```python
from build123d import *

# Parameters (mm, degrees)
F1_DEPTH = 7.2


with BuildPart() as f1:
    # F0 (on Top) → F1 (new body)
    with BuildSketch(Plane.XY):
        with BuildLine():
            Line((-8.2668317482, -17.3311792314), (0.1017643333, -17.3311792314))
            Line((0.1017643333, -17.3311792314), (8.2668317482, -17.3311792314))
            add(Edge.make_bspline(
                [(36.6192528714, -21.1421355028), (36.0259011039, -22.4667622734), (33.1013576776, -26.9667648317), (23.9156707234, -28.3936125615), (14.039303545, -21.4118387937), (8.2668317482, -17.3311792314)],
                knots=[0.4597765415, 0.4597765415, 0.4597765415, 0.4597765415, 0.5296754291, 0.7251078993, 1, 1, 1, 1], degree=3))
            add(Edge.make_bspline(
                [(36.6192528714, -21.1421355028), (37.4697374215, -19.9659644134), (39.9045822409, -15.1832342327), (36.5474251452, -6.5147721142), (25.5628481096, -1.4524741246), (19.142657366, 1.506303313)],
                knots=[0.4597765415, 0.4597765415, 0.4597765415, 0.4597765415, 0.5296754291, 0.7251078993, 1, 1, 1, 1], degree=3))
            Line((19.142657366, 1.506303313), (10.8758256178, 15.8248759184))
            add(Edge.make_bspline(
                [(0, 42.2842710057), (1.4438363177, 42.4327266869), (6.8032245633, 42.1499990644), (12.6317544218, 34.9083846758), (11.5235445645, 22.8643129183), (10.8758256178, 15.8248759184)],
                knots=[0.4597765415, 0.4597765415, 0.4597765415, 0.4597765415, 0.5296754291, 0.7251078993, 1, 1, 1, 1], degree=3))
            add(Edge.make_bspline(
                [(0, 42.2842710057), (-1.4438363177, 42.4327266869), (-6.8032245633, 42.1499990644), (-12.6317544218, 34.9083846758), (-11.5235445645, 22.8643129183), (-10.8758256178, 15.8248759184)],
                knots=[0.4597765415, 0.4597765415, 0.4597765415, 0.4597765415, 0.5296754291, 0.7251078993, 1, 1, 1, 1], degree=3))
            Line((-10.8758256178, 15.8248759184), (-19.142657366, 1.506303313))
            add(Edge.make_bspline(
                [(-36.6192528714, -21.1421355028), (-37.4697374215, -19.9659644134), (-39.9045822409, -15.1832342327), (-36.5474251452, -6.5147721142), (-25.5628481096, -1.4524741246), (-19.142657366, 1.506303313)],
                knots=[0.4597765415, 0.4597765415, 0.4597765415, 0.4597765415, 0.5296754291, 0.7251078993, 1, 1, 1, 1], degree=3))
            add(Edge.make_bspline(
                [(-36.6192528714, -21.1421355028), (-36.0259011039, -22.4667622734), (-33.1013576776, -26.9667648317), (-23.9156707234, -28.3936125615), (-14.039303545, -21.4118387937), (-8.2668317482, -17.3311792314)],
                knots=[0.4597765415, 0.4597765415, 0.4597765415, 0.4597765415, 0.5296754291, 0.7251078993, 1, 1, 1, 1], degree=3))
        make_face()
        Polygon((-31.2220487017, -10.6943638675), (-24.8726151374, -5.881392497), (-17.5297428808, -8.9736775782), (-17.3953376506, -10.0432028752), (-16.5363041885, -16.8789340297), (-22.8857377528, -21.6919054001), (-30.2286100094, -18.599620319), align=None, mode=Mode.SUBTRACT)
        with BuildLine():
            ThreePointArc((0.0640009602, -10.8998121028), (-9.9190071048, 4.5192143183), (8.2668317482, 7.1041884017))
            add(Edge.make_bspline(
                [(8.2668317482, 7.1041884017), (8.6052555966, 6.6408728417), (8.943679445, 6.1775572816), (9.2821032933, 5.7142417215)],
                knots=[0, 0, 0, 0, 1.7212577042, 1.7212577042, 1.7212577042, 1.7212577042], degree=3))
            ThreePointArc((9.2821032933, 5.7142417215), (9.5312177763, -5.2882783305), (0.0640009602, -10.8998121028))
        make_face(mode=Mode.SUBTRACT)
        Polygon((24.8726151374, -21.6919054001), (17.5297428808, -18.599620319), (16.5363041884, -10.6943638675), (17.3953376506, -10.0432028752), (22.8857377528, -5.881392497), (30.2286100094, -8.9736775782), (31.2220487017, -16.8789340297), (30.3630152395, -17.5300950219), align=None, mode=Mode.SUBTRACT)
        Polygon((-6.3494335643, 32.3862692676), (0.9934386923, 35.4785543487), (7.3428722566, 30.6655829783), (6.3494335643, 22.7603265268), (0, 20.0864057505), (-0.9934386923, 19.6680414456), (-7.3428722566, 24.481012816), align=None, mode=Mode.SUBTRACT)
    extrude(amount=F1_DEPTH)


solid = f1.part
```
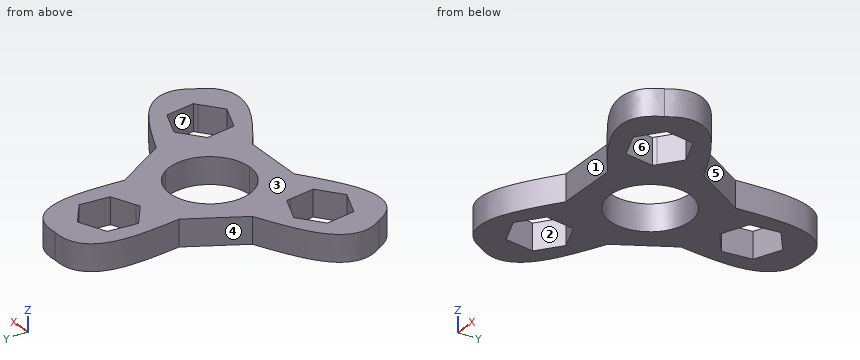
Verification items for the finished model (mm, model axes). Face numbers are marked on the shaded views. A direction names the side the tool comes from. Round coordinates to 2 decimals unless told otherwise and drop trailing zeros. Write each loop counter-clockwise with the first axis right and the second up, starting at its lowest first coordinate (ties: lowest second). Pieces come first, ordered by that corner, then holes. Notation, with made-up numbers: (54, 54.25) - (62, 54.25) arc R29 ccw to (62, 82.25) - close; hole circle Ø1 at (-7, 88). An arc over 180 degrees is marked (long way). Answer as a JSON object with one key per item and string values. Group by question number.
Q1. Tool access check on the marked faces 1, 2 and 3. Record the directions out of +Z, -Z, +X, -X, +Y, -Y that give a thin tool (end or side, any length) a straight path to the whole face; none if there is none.
Q2. Section check A-A, the plane y = 4. Enter the section's corners in (x, z), plus the area to 3 significant figures.
Q3. Thickness scan on line 1 (Y direction, x = 0, z = 5.75); line 2 (X direction, y = -10, z = 2.5); line 3 (X direction, y = -8, z = 1.5). Record the ranges inside material, lowest first.
Q4. Mould release check, pull along X, two halves, no side actions. Record for the marked faces 4, 5, 6 and 7: released by +X, released by -X, zero draft, split by the parting line, or undercut.
Q5. Go/stop test with flat-tipped pins: pin 1 Ø2 at (x, z) = (-25.5, 5.5) entering from +Y; pin 2 Ø3 at (y, z) = (32.5, 1.5) entering from -X; pin 3 Ø3 at (y, z) = (32.5, 1.5) entering from +X. Record where each tip stops, or that it passes through.
Q6. Section check B-B, the plane z = 6. Give the number of separate pieces and of enclosed holes in the cut face, plus the area to 3 significant figures.
Found:
{
 "1": {"face 1": "+Z, -Z, -Y", "face 2": "+Z, -Z", "face 3": "+Z, +X, -X, +Y, -Y"},
 "2": {"outline": "(-17.7, 0) - (-10.14, 0) - (-10.14, 7.2) - (-17.7, 7.2) - close; (10.14, 0) - (17.7, 0) - (17.7, 7.2) - (10.14, 7.2) - close", "area": "109 mm^2"},
 "3": {"line 1": "y = -17.33 to -10.9, 10.9 to 20.09, 35.06 to 42.28", "line 2": "x = -37.11 to -30.31, -17.4 to -4.34, 4.34 to 17.45, 30.36 to 37.11", "line 3": "x = -35.43 to -27.67, -19.84 to -7.4, 7.4 to 20.09, 27.92 to 35.43"},
 "4": {"face 4": "released by -X", "face 5": "released by +X", "face 6": "undercut", "face 7": "undercut"},
 "5": {"pin 1": "stops at y = -1.01", "pin 2": "stops at x = -11.43", "pin 3": "stops at x = 11.43"},
 "6": {"separate pieces": "1", "enclosed holes": "4", "area": "1,750 mm^2"}
}
